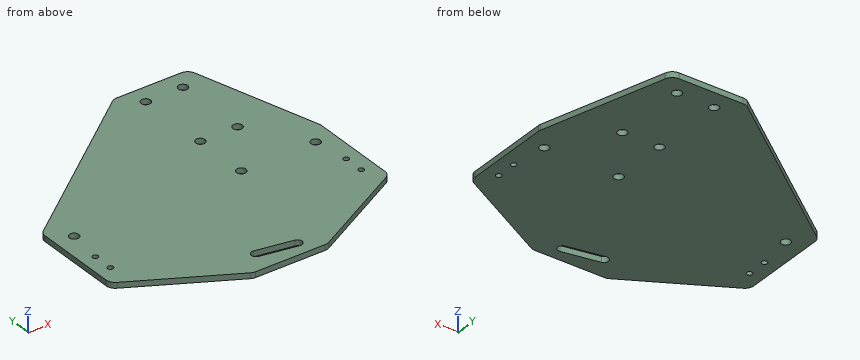
```python
from build123d import *

# Parameters (mm, degrees)
BOSS_EXTRUDE1_DEPTH  = 3
SKETCH2_R            = 2.5
SKETCH2_R_2          = 1.5
CUT_EXTRUDE1_DEPTH   = 4
SKETCH3_R            = 2.5
CUT_EXTRUDE2_DEPTH   = 4
LPATTERN1_COUNT      = 2
LPATTERN1_PITCH      = 20
LPATTERN1_COUNT_DIR2 = 2
LPATTERN1_PITCH_DIR2 = 40
CUT_EXTRUDE3_DEPTH   = 4
FILLET1_R            = 5


with BuildPart() as part:
    # Sketch1 → Boss-Extrude1 (new body)
    with BuildSketch(Plane.XY):
        Polygon((-75, 0), (-75, 80), (15, 150), (55, 150), (75, 80), (75, 0), align=None)
    extrude(amount=BOSS_EXTRUDE1_DEPTH)

    # Sketch2 → Cut-Extrude1 (cut, through all)
    with BuildSketch(Plane.XY.offset(3)):
        with Locations((-65, 70)):
            Circle(SKETCH2_R)
        with Locations((65, 70)):
            Circle(SKETCH2_R)
        with Locations((67.5, 51)):
            Circle(SKETCH2_R_2)
        with Locations((25, 70)):
            Circle(SKETCH2_R)
        with Locations((67.5, 40)):
            Circle(SKETCH2_R_2)
        with Locations((-67.5, 51)):
            Circle(SKETCH2_R_2)
        with Locations((-67.5, 40)):
            Circle(SKETCH2_R_2)
        with BuildLine():
            Line((-9.413957086, 14.198501159), (10.282197974, 10.725537606))
            ThreePointArc((10.282197974, 10.725537606), (12.310096913, 7.829397779), (9.413957086, 5.801498841))
            Line((9.413957086, 5.801498841), (-10.282197974, 9.274462394))
            ThreePointArc((-10.282197974, 9.274462394), (-12.310096913, 12.170602221), (-9.413957086, 14.198501159))
        make_face()
    extrude(amount=-CUT_EXTRUDE1_DEPTH, mode=Mode.SUBTRACT)

    # Sketch3 → Cut-Extrude2 (cut, through all)
    with BuildSketch(Plane.XY.offset(3)):
        with Locations((45, 140)):
            Circle(SKETCH3_R)
    cut_extrude2 = extrude(amount=-CUT_EXTRUDE2_DEPTH, mode=Mode.SUBTRACT)

    # LPattern1: Cut-Extrude2 2 × 2
    with Locations(*[(-i * LPATTERN1_PITCH, -j * LPATTERN1_PITCH_DIR2, 0) for i in range(LPATTERN1_COUNT) for j in range(LPATTERN1_COUNT_DIR2) if (i, j) != (0, 0)]):
        add(cut_extrude2, mode=Mode.SUBTRACT)

    # Sketch4 → Cut-Extrude3 (cut, through all)
    with BuildSketch(Plane.XY.offset(3)):
        Polygon((-75, 30), (-20, 0), (-75, 0), align=None)
        Polygon((20, 0), (75, 30), (75, 0), align=None)
    extrude(amount=-CUT_EXTRUDE3_DEPTH, mode=Mode.SUBTRACT)

    # Fillet1
    fillet1_edges = [part.edges().sort_by_distance(p)[0] for p in [
        (55, 150, 1.5),
        (75, 80, 1.5),
        (-75, 80, 1.5),
        (15, 150, 1.5),
        (-75, 30, 1.5),
        (-20, 0, 1.5),
        (20, 0, 1.5),
        (75, 30, 1.5),
    ]]
    fillet(fillet1_edges, radius=FILLET1_R)


solid = part.part
```
For this review, take the finished solid that the model builds, in its own axes (mm). Round coordinates to 2 decimals unless told otherwise and drop trailing zeros. Order: outer loops, then holes, each group sorted by start corner. A loop starts at its lowest first (then second) coordinate and runs counter-clockwise, first axis right, second up.
Q1. Insertion check: P1, Ø4.5, axis at x = 25, y = 70, coming from the +Z side. The pin has a flat end and moves straight along its axis. Give the tip position at first contact, or say it passes through.
Findings below:
P1: passes through
Q2. We need section D-D, the plane x = -25. Give the boundary of the cut face in (y, z), plus the area to 3 significant figures.
Findings below:
outline: (2.73, 0) - (118.89, 0) - (118.89, 3) - (2.73, 3) - close
area: 348 mm2
Q3. We need section A-A, the plane y = 70. Give the boundary of the cut face in (x, z).
Findings below:
outline: (-75, 0) - (-67.5, 0) - (-67.5, 3) - (-75, 3) - close; (-62.5, 0) - (22.5, 0) - (22.5, 3) - (-62.5, 3) - close; (27.5, 0) - (62.5, 0) - (62.5, 3) - (27.5, 3) - close; (67.5, 0) - (75, 0) - (75, 3) - (67.5, 3) - close
Q4. Wall thickness on line 1 (Y direction, x = 45, z = 1.8); line 2 (Y direction, x = 25, z = 1.05); line 3 (Y direction, x = 27, z = 0.75): over which ranges is each line inside the solid? List them lowest first.
Findings below:
line 1: y = 13.64 to 97.5, 102.5 to 137.5, 142.5 to 150
line 2: y = 2.73 to 67.5, 72.5 to 97.5, 102.5 to 137.5, 142.5 to 150
line 3: y = 3.82 to 68.5, 71.5 to 98.5, 101.5 to 138.5, 141.5 to 150
Q5. We need section B-B, the plane z = 1.95. State how many separate pieces and enclosed holes the cut face has, plus the area to 3 significant figures.
Findings below:
separate pieces: 1
enclosed holes: 12
area: 16,700 mm2
Q6. We need section C-C, the plane y = 140. Give the boundary of the cut face in (x, z), plus the area to 3 significant figures.
Findings below:
outline: (2.14, 0) - (22.5, 0) - (22.5, 3) - (2.14, 3) - close; (27.5, 0) - (42.5, 0) - (42.5, 3) - (27.5, 3) - close; (47.5, 0) - (57.86, 0) - (57.86, 3) - (47.5, 3) - close
area: 137 mm2
